```python
from build123d import *

# Parameters (mm, degrees)
SKETCH1_W           = 40
SKETCH1_H           = 43
SKETCH1_R           = 2
BOSS_EXTRUDE1_DEPTH = 4
SKETCH4_W           = 40
SKETCH4_H           = 3
BOSS_EXTRUDE2_DEPTH = 40
SKETCH5_R           = 6.75
CUT_EXTRUDE5_DEPTH  = 34
SKETCH8_R           = 1.5
CUT_EXTRUDE6_DEPTH  = 10
BOSS_EXTRUDE3_DEPTH = 2
BOSS_EXTRUDE4_DEPTH = 2


with BuildPart() as part:
    # Sketch1 → Boss-Extrude1 (new body)
    with BuildSketch(Plane(origin=(0, 0, 0), x_dir=(1, 0, 0), z_dir=(0, 1, 0))):
        Rectangle(SKETCH1_W, SKETCH1_H)
        with Locations(Location((-14.715053003, 12, 0), (0, 0, 270))):
            Circle(SKETCH1_R, mode=Mode.SUBTRACT)
        with Locations(Location((15.284946997, 12, 0), (0, 0, 270))):
            Circle(SKETCH1_R, mode=Mode.SUBTRACT)
        with Locations(Location((-14.715053003, -12, 0), (0, 0, 270))):
            Circle(SKETCH1_R, mode=Mode.SUBTRACT)
        with Locations(Location((15.284946997, -12, 0), (0, 0, 270))):
            Circle(SKETCH1_R, mode=Mode.SUBTRACT)
    extrude(amount=-BOSS_EXTRUDE1_DEPTH)

    # Sketch4 → Boss-Extrude2 (add)
    with BuildSketch(Plane(origin=(0, 0, 0), x_dir=(1, 0, 0), z_dir=(0, 1, 0))):
        with Locations((0, 20)):
            Rectangle(SKETCH4_W, SKETCH4_H)
    extrude(amount=BOSS_EXTRUDE2_DEPTH)

    # Sketch5 → Cut-Extrude5 (cut)
    with BuildSketch(Plane.XY.offset(-18.5)):
        with Locations((0, 25)):
            Circle(SKETCH5_R)
    extrude(amount=-CUT_EXTRUDE5_DEPTH, mode=Mode.SUBTRACT)

    # Sketch8 → Cut-Extrude6 (cut)
    with BuildSketch(Plane.XY.offset(-18.5)):
        with Locations((-15.5, 18)):
            Circle(SKETCH8_R)
        with Locations((-9.049038106, 30.673393759)):
            Circle(SKETCH8_R)
        with Locations((5.151923789, 31.423393759)):
            Circle(SKETCH8_R)
        with Locations((12.901923789, 19.5)):
            Circle(SKETCH8_R)
        with Locations((6.450961894, 6.826606241)):
            Circle(SKETCH8_R)
        with Locations((-7.75, 6.076606241)):
            Circle(SKETCH8_R)
    extrude(amount=-CUT_EXTRUDE6_DEPTH, mode=Mode.SUBTRACT)

    # Sketch9 → Boss-Extrude3 (add)
    with BuildSketch(Plane(origin=(20, 0, 0), x_dir=(0, 0, -1), z_dir=(1, 0, 0))):
        Polygon((18.5, 13), (3.5, 0), (18.5, 0), align=None)
    extrude(amount=-BOSS_EXTRUDE3_DEPTH)

    # Sketch10 → Boss-Extrude4 (add)
    with BuildSketch(Plane.ZY.offset(20)):
        Polygon((-18.5, 13), (-3.5, 0), (-18.5, 0), align=None)
    extrude(amount=-BOSS_EXTRUDE4_DEPTH)


solid = part.part
```
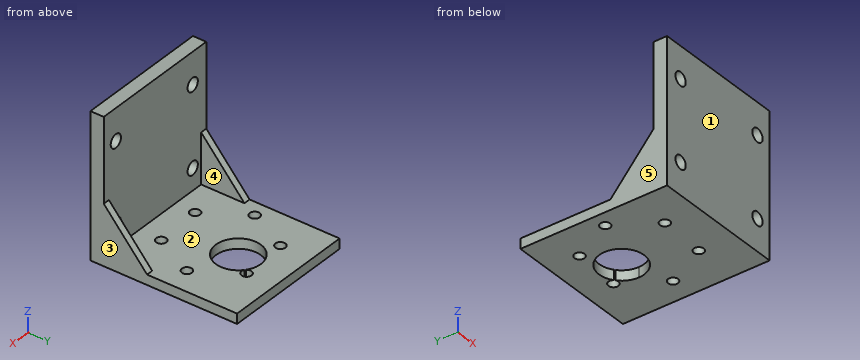
CAD build for the part. Positions are in the model's coordinates, mm. Face numbers are marked on the shaded views. A direction names the side the tool comes from. Coordinates: 2 decimals unless noted, no trailing zeros. Order: outer loops, then holes, each group sorted by start corner. A loop starts at its lowest first (then second) coordinate and runs counter-clockwise, first axis right, second up. Notation, with made-up numbers: M -31,60 L -19,60 A15 cw -19,67 Z; hole C 71,-23.75 d4. An arc over 180 degrees is marked long. Answer as CSV lines item,"result".
1) Cut at D-D (y = 15.5). List the corners of the cut face in (x, z).
Verdict:
outline,"M -20,-21.5 L 20,-21.5 L 20,-18.5 L -20,-18.5 Z"
2) Drill centre lines: L1, parallel to Y at x = -15.5, z = -20.15; L2, parallel to X at y = 5.5, z = -17.5; L3, parallel to Y at x = 14.5, z = 7. Where is each one in solid material? Low to high. Write a range as from..to.
Verdict:
L1,"-4..16.5, 19.5..40"
L2,"-20..-18, 18..20"
L3,"-4..0"
3) Cut at B-B (z = -11). List the corners of the cut face in (x, y).
Verdict:
outline,"M -20,-4 L -16.45,-4 L -16.45,0 L -18,0 L -18,6.5 L -20,6.5 Z; M -12.98,-4 L 13.55,-4 L 13.55,0 L -12.98,0 Z; M 17.02,-4 L 20,-4 L 20,6.5 L 18,6.5 L 18,0 L 17.02,0 Z"
4) Cut at C-C (x = -15.5). List the corners of the cut face in (y, z).
Verdict:
outline,"M -4,-21.5 L 16.5,-21.5 L 16.5,-18.5 L 0,-18.5 L 0,-13.84 L -4,-13.84 Z; M -4,-10.16 L 0,-10.16 L 0,10.16 L -4,10.16 Z; M -4,13.84 L 0,13.84 L 0,21.5 L -4,21.5 Z; M 19.5,-21.5 L 40,-21.5 L 40,-18.5 L 19.5,-18.5 Z"
5) 3-axis set-ups, long thin cutter, end or side, ignore diameter. For the marked faces 1 and 2: which of +Z, -Z, +X, -X, +Y, -Y reach the whole face in a straight line?
Verdict:
face 1,"+Z, -Z, +X, -X, -Y"
face 2,"+Z, +Y"
6) Mould opens along X. For the marked faces 3, 4 and 5 say: released by +X, released by -X, zero draft, split by the parting line, or undercut.
Verdict:
face 3,"released by +X"
face 4,"undercut"
face 5,"released by -X"
7) Flat gauge pins, fed straight in: P1, Ø2.5, axis at x = -9.05, y = 30.67, coming from the -Z side; P2, Ø4, axis at x = 5.15, y = 31.42, coming from the +Z side; P3, Ø12, axis at x = 2, z = -4, coming from the +Y side. Where does each tip first touch, or does it go through?
Verdict:
P1,"through"
P2,"z = -18.5"
P3,"y = 0"
8) Cut at A-A (x = 0). List the corners of the cut face in (y, z).
Verdict:
outline,"M -4,-21.5 L 18.25,-21.5 L 18.25,-18.5 L 0,-18.5 L 0,21.5 L -4,21.5 Z; M 31.75,-21.5 L 40,-21.5 L 40,-18.5 L 31.75,-18.5 Z"
